Job drawing, mm, ordinate dimensions from the low corner. One solid piece. Give positions to 0.01 mm unless a question says otherwise; leave off trailing zeros. Order: outer loops, then holes, each group sorted by start corner. A loop starts at its lowest first (then second) coordinate and runs counter-clockwise, first axis right, second up. Notation, with made-up numbers: (63, -25.75) - (78, -25.75) arc R24 cw to (78, 10.25) - close; hole circle Ø8 at (34, 77.5). An arc over 180 degrees is marked (long way). Use a Markdown table: item, result. Add a question column.
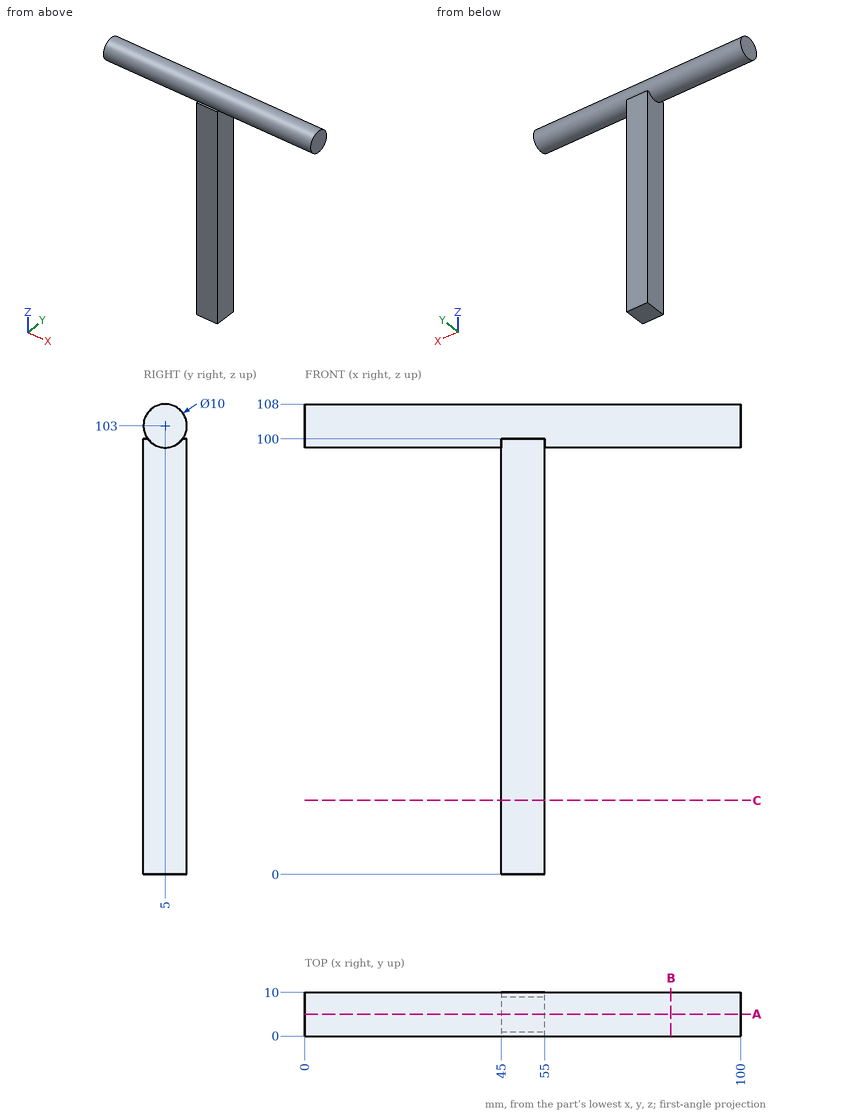
1. Pin check, flat tips, straight feed: P1, Ø1, axis at y = 4.5, z = 33, coming from the +X side; P2, Ø0.5, axis at x = 49, y = 0.5, coming from the +Z side; P3, Ø2, axis at x = 58.5, y = 3, coming from the -Z side. Stop position of each tip, or through.
2. Cut at C-C (z = 17). Write the cut outline in (x, y).
3. Drill centre lines: probe 1 along X at (y, z) = (4.5, 89.5); probe 2 along Z at (x, y) = (59.5, 5.25); probe 3 along Z at (x, y) = (26, 2). Where is each one in solid material? Low to high. Write a range as [from, to].
4. Cut at A-A (y = 5). Write the cut outline in (x, z), plus the area to 3 significant figures.
5. Cut at B-B (x = 84). Write the cut outline in (y, z), plus the area to 3 significant figures.
Responses:
| question | item | result |
|---|---|---|
| 1 | P1 | stops at x = 55 |
| 1 | P2 | stops at z = 105.63 |
| 1 | P3 | stops at z = 98.1 |
| 2 | outline | (45, 0) - (55, 0) - (55, 10) - (45, 10) - close |
| 3 | probe 1 | x = [45, 55] |
| 3 | probe 2 | z = [98.01, 107.99] |
| 3 | probe 3 | z = [99, 107] |
| 4 | outline | (0, 98) - (45, 98) - (45, 0) - (55, 0) - (55, 98) - (100, 98) - (100, 108) - (0, 108) - close |
| 4 | area | 1,980 mm² |
| 5 | outline | circle Ø10 at (5, 103) |
| 5 | area | 78.5 mm² |
